Can you work these out from the model? Positions are in its coordinate system, mm. Face numbers are marked on the shaded views. A direction names the side the tool comes from. Give positions to 0.01 mm unless a question says otherwise; leave off trailing zeros. Write each loop counter-clockwise with the first axis right and the second up, starting at its lowest first coordinate (ties: lowest second). Pieces come first, ordered by that corner, then holes.
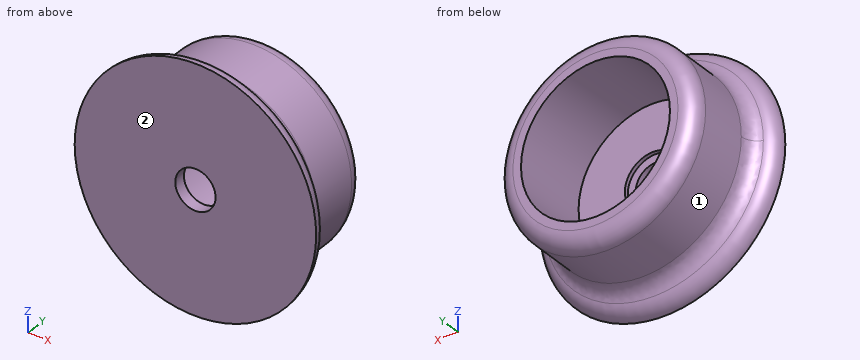
Autodesk Inventor part; units mm, degrees
ref_plane "YZ Plane" through (0, 0, 0) normal (1, 0, 0) x (0, 1, 0)
ref_plane "XZ Plane" through (0, 0, 0) normal (0, 1, 0) x (-1, 0, 0)
ref_plane "XY Plane" through (0, 0, 0) normal (0, 0, 1) x (1, 0, 0)
sketch "Sketch1" plane through (0, 0, 0) normal (0, 1, 0) x (-1, 0, 0)
  circle A0 centre (0, 0) radius 9.25
  circle A1 centre (0, 0) radius 12.25
  dimension "d0" = 18.5
  dimension "d1" = 24.5
extrude "Extrusion1" add sketch "Sketch1" along normal blind 10
fillet "Fillet1" radius 2 1 edges at (12.25, 10, 0)
sketch "Sketch2" plane through (0, 0, 0) normal (0, -1, 0) x (1, 0, 0)
  circle A0 centre (0, 0) radius 9.25
  circle A1 centre (0, 0) radius 12.25
  circle A2 centre (0, 0) radius 15
  circle A3 centre (0, 0) radius 2.5
  dimension "d6" = 30
  dimension "d9" = 5
extrude "Extrusion2" add sketch "Sketch2" along normal blind 2 contours A0 | A1 | A2
fillet "Fillet3" radius 2 2 edges at (-15, 0, 0) (12.25, 0, 0)
sketch "Sketch3" plane through (0, 0, 0) normal (0, 1, 0) x (1, 0, 0)
  circle A0 centre (0, 0) radius 2.5
  circle A1 centre (0, 0) radius 9.25
  circle A2 centre (0, 0) radius 3.5
  dimension "d12" = 7
extrude "Extrusion3" cut sketch "Sketch3" against normal blind 0.5 contours A2
equation "\"BendRadius\" = Thickness"
equation "\"BendReliefWidth\" = Thickness"
equation "\"BendReliefDepth\" = 0.5 * Thickness"
equation "\"CornerReliefSize\" = 4 * Thickness"
equation "\"MinimumRemnant\" = 2 * Thickness"
equation "\"TransitionRadius\" = BendRadius"
equation "\"JacobiRadiusSize\" = BendRadius"
equation "\"GapSize\" = Thickness"
properties part number "powerButtonPart2"
(1) Imagine slicing it at B-B, the plane y = 9. Write out the boundary of the cut face in (x, z), plus the area to 3 significant figures.
Returned:
outline: circle Ø23.96 at (0, 0); hole circle Ø18.5 at (0, 0)
area: 182 mm2
(2) For the marked faces 1 and 2, which set-ups out of +Z, -Z, +X, -X, +Y, -Y let a thin tool reach every point of the face, with its end or its side?
Returned:
face 1: +Y
face 2: +Z, -Z, +X, -X, -Y
(3) If I drill on L1, parallel to X at y = 6.75, z = -6; L2, parallel to X at y = 4.25, z = -7; L3, parallel to Z at x = -5.5, y = 7.5, over which ranges is the centre line in solid material (lowest first)?
Returned:
L1: x = -10.68 to -7.04, 7.04 to 10.68
L2: x = -10.05 to -6.05, 6.05 to 10.05
L3: z = -10.95 to -7.44, 7.44 to 10.95
(4) Will these pins go through, and if not, where does the flat tip stop? P1, Ø9, axis at x = -3.5, z = 3, coming from the +Y side; P2, Ø2, axis at y = 8, z = -2.5, coming from the +X side; P3, Ø2, axis at x = 1, z = -1.5, coming from the +Y side.
Returned:
P1: stops at y = 0
P2: stops at x = 12.16
P3: stops at y = -0.5
(5) Imagine slicing it at A-A, the plane y = 3.25. Write out the boundary of the cut face in (x, z).
Returned:
outline: circle Ø24.5 at (0, 0); hole circle Ø18.5 at (0, 0)
